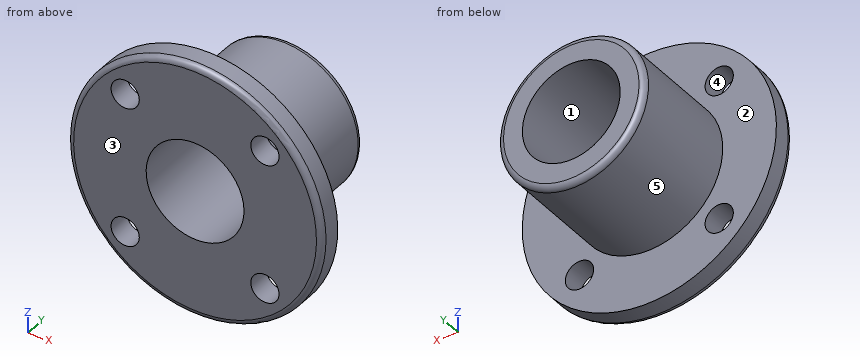
from build123d import *

# Parameters (mm, degrees)
SKETCH1_R                       = 28.575
BOSS_EXTRUDE1_DEPTH             = 5.08
SKETCH2_R                       = 16.51
BOSS_EXTRUDE2_DEPTH             = 25.4
F_1_4_0_25_DIAMETER_HOLE1_D     = 6.35
F_1_4_0_25_DIAMETER_HOLE1_DEPTH = 8.89
F_1_4_0_25_DIAMETER_HOLE1_TIP   = 1.907732465
CUT_EXTRUDE1_DEPTH              = 51.617108274
CUT_EXTRUDE1_DEPTH_BACK         = 51.617108274
SKETCH5_R                       = 11
FILLET1_R                       = 1.27


with BuildPart() as part:
    # Sketch1 → Boss-Extrude1 (new body)
    with BuildSketch(Plane(origin=(0, 0, 0), x_dir=(1, 0, 0), z_dir=(0, 1, 0))):
        with Locations(Location((0, 0, 0), (0, 0, 270))):
            Circle(SKETCH1_R)
    extrude(amount=BOSS_EXTRUDE1_DEPTH)

    # Sketch2 → Boss-Extrude2 (add)
    with BuildSketch(Plane(origin=(0, 5.08, 0), x_dir=(1, 0, 0), z_dir=(0, 1, 0))):
        with Locations(Location((0, 0, 0), (0, 0, 270))):
            Circle(SKETCH2_R)
    extrude(amount=BOSS_EXTRUDE2_DEPTH)

    # 1/4 (0.25) Diameter Hole1
    with Locations(Plane(origin=(0, 0, 0), x_dir=(-1, 0, 0), z_dir=(0, -1, 0))):
        with Locations((15.715448212, 15.715448212), (-15.715448212, 15.715448212), (-15.715448212, -15.715448212), (15.715448212, -15.715448212)):
            Hole(F_1_4_0_25_DIAMETER_HOLE1_D / 2, depth=F_1_4_0_25_DIAMETER_HOLE1_DEPTH)
            with Locations((0, 0, -(F_1_4_0_25_DIAMETER_HOLE1_DEPTH + F_1_4_0_25_DIAMETER_HOLE1_TIP / 2))):  # 118° drill point
                Cone(0, F_1_4_0_25_DIAMETER_HOLE1_D / 2, F_1_4_0_25_DIAMETER_HOLE1_TIP, mode=Mode.SUBTRACT)

    # Sketch5 → Cut-Extrude1 (cut, two sides: drawn at the far end of the back side and taken through both)
    with BuildSketch(Plane(origin=(0, 30.48, 0), x_dir=(1, 0, 0), z_dir=(0, 1, 0)).offset(-CUT_EXTRUDE1_DEPTH_BACK)):
        with Locations(Location((0, 0, 0), (0, 0, 270))):
            Circle(SKETCH5_R)
    extrude(amount=CUT_EXTRUDE1_DEPTH + CUT_EXTRUDE1_DEPTH_BACK, mode=Mode.SUBTRACT)

    # Fillet1
    fillet1_edges = [part.edges().sort_by_distance(p)[0] for p in [
        (0, 0, -28.575),
        (0, 30.48, -16.51),
    ]]
    fillet(fillet1_edges, radius=FILLET1_R)


solid = part.part
CAD build for the part. Positions are in the model's coordinates, mm. Face numbers are marked on the shaded views. A direction names the side the tool comes from. Give positions to 0.01 mm unless a question says otherwise; leave off trailing zeros. Write each loop counter-clockwise with the first axis right and the second up, starting at its lowest first coordinate (ties: lowest second). Pieces come first, ordered by that corner, then holes. Notation, with made-up numbers: (-14, 40.5) - (-2, 40.5) arc R22 ccw to (-2, 68.5) - close; hole circle Ø8 at (-29.75, 68). An arc over 180 degrees is marked (long way). Answer as CSV lines item,"result".
Q1. Drill centre lines: line 1 (X direction, y = 18, z = 0); line 2 (Z direction, x = -2, y = 9.5); line 3 (X direction, y = 6.5, z = -8.5). Where is each one in solid material? Low to high. Write a range as from..to.
Result set:
line 1,"-16.51..-11, 11..16.51"
line 2,"-16.39..-10.82, 10.82..16.39"
line 3,"-14.15..-6.98, 6.98..14.15"
Q2. 3-axis set-ups, long thin cutter, end or side, ignore diameter. For the marked faces 1 and 2: which of +Z, -Z, +X, -X, +Y, -Y reach the whole face in a straight line?
Result set:
face 1,"+Y, -Y"
face 2,"+Y"
Q3. Band-saw the part on C-C (y = 22.5). Give the cut face in (x, z), and give its area (3 significant figures).
Result set:
outline,"circle Ø33.02 at (0, 0); hole circle Ø22 at (0, 0)"
area,"476 mm²"
Q4. Band-saw the part on D-D (x = -14.5). State how many separate pieces and enclosed holes the cut face has, and give its area (3 significant figures).
Result set:
separate pieces,"3"
enclosed holes,"0"
area,"589 mm²"
Q5. Band-saw the part on A-A (x = 0). Give the cut face in (y, z) (3 decimals), and give its area (3 significant figures).
Result set:
outline,"(0, -27.305) arc R1.27 ccw to (1.27, -28.575) - (5.08, -28.575) - (5.08, -16.51) - (29.21, -16.51) arc R1.27 ccw to (30.48, -15.24) - (30.48, -11) - (0, -11) - close; (0, 11) - (30.48, 11) - (30.48, 15.24) arc R1.27 ccw to (29.21, 16.51) - (5.08, 16.51) - (5.08, 28.575) - (1.27, 28.575) arc R1.27 ccw to (0, 27.305) - close"
area,"457 mm²"
Q6. Flat gauge pins, fed straight in: pin 1 Ø4 at (x, z) = (-15.72, 15.72) entering from -Y; pin 2 Ø12 at (x, y) = (2.5, 25.5) entering from -Z; pin 3 Ø2 at (y, z) = (4, 22.5) entering from -X; pin 4 Ø8 at (y, z) = (23.5, -11) entering from +X. Where does each tip first touch, or does it go through?
Result set:
pin 1,"through"
pin 2,"z = -16.51"
pin 3,"x = -18.82"
pin 4,"x = 14.95"
Q7. Pull direction Z, two halves, no side cores. Call the marked faces 3, 4 and 5: released by +Z, released by -Z, zero draft, split by the parting line, or undercut.
Result set:
face 3,"zero draft"
face 4,"undercut"
face 5,"split by the parting line"
Q8. Band-saw the part on B-B (z = 0). Give the cut face in (x, y) (3 decimals), and give its area (3 significant figures).
Result set:
outline,"(-28.575, 1.27) arc R1.27 ccw to (-27.305, 0) - (-11, 0) - (-11, 30.48) - (-15.24, 30.48) arc R1.27 ccw to (-16.51, 29.21) - (-16.51, 5.08) - (-28.575, 5.08) - close; (11, 0) - (27.305, 0) arc R1.27 ccw to (28.575, 1.27) - (28.575, 5.08) - (16.51, 5.08) - (16.51, 29.21) arc R1.27 ccw to (15.24, 30.48) - (11, 30.48) - close"
area,"457 mm²"
